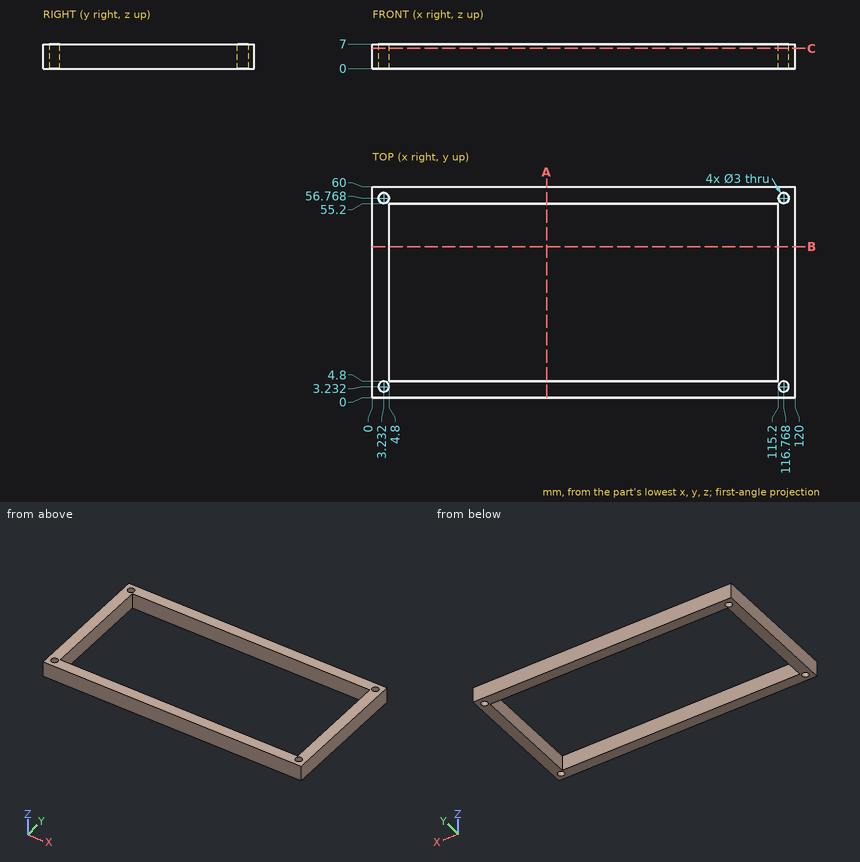
Input: dimensioned drawing with shaded views. Units: mm. Origin: part minimum x, y, z. Give positions to 0.01 mm unless a question says otherwise; leave off trailing zeros. Write each loop counter-clockwise with the first axis right and the second up, starting at its lowest first coordinate (ties: lowest second). Pieces come first, ordered by that corner, then holes. Notation, with made-up numbers: (78, 48) -> (93, 48) arc R4 ccw to (93, 55) -> close; hole circle Ø5 at (-28.75, 87). An arc over 180 degrees is marked (long way). Answer as a JSON object with one key per item and string values.
1. Cut plane C-C on z = 5.75. Output: boundary loops of the cut face in (x, y), and give its area (3 significant figures).
Ans:
{"outline": "(0, 0) -> (120, 0) -> (120, 60) -> (0, 60) -> close; hole circle Ø3 at (3.23, 3.23); hole circle Ø3 at (3.23, 56.77); hole (4.8, 4.8) -> (115.2, 4.8) -> (115.2, 55.2) -> (4.8, 55.2) -> close; hole circle Ø3 at (116.77, 3.23); hole circle Ø3 at (116.77, 56.77)", "area": "1,610 mm^2"}
2. Cut plane A-A on x = 49.5. Output: boundary loops of the cut face in (y, z), and give its area (3 significant figures).
Ans:
{"outline": "(0, 0) -> (4.8, 0) -> (4.8, 7) -> (0, 7) -> close; (55.2, 0) -> (60, 0) -> (60, 7) -> (55.2, 7) -> close", "area": "67.2 mm^2"}
3. Cut plane B-B on y = 43. Output: boundary loops of the cut face in (x, z).
Ans:
{"outline": "(0, 0) -> (4.8, 0) -> (4.8, 7) -> (0, 7) -> close; (115.2, 0) -> (120, 0) -> (120, 7) -> (115.2, 7) -> close"}
4. Ray query, probe 1 along Y at (x, z) = (110.5, 6.75); probe 2 along X at (y, z) = (11.5, 6.75); probe 3 along X at (y, z) = (56, 6). Return the intervals inside material, ascending. Write a range as from..to.
Ans:
{"probe 1": "y = 0..4.8, 55.2..60", "probe 2": "x = 0..4.8, 115.2..120", "probe 3": "x = 0..1.94, 4.52..115.48, 118.06..120"}
